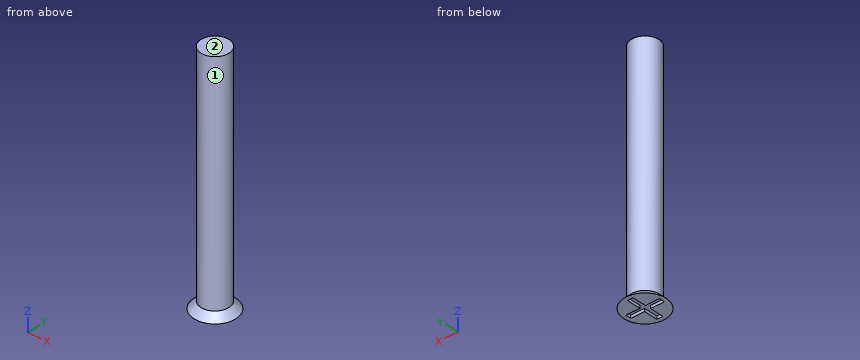
from build123d import *

# Parameters (mm, degrees)
SKETCH1_R           = 0.5
BOSS_EXTRUDE1_DEPTH = 4.1
CUT_EXTRUDE1_DEPTH  = 0.1


with BuildPart() as part:
    # Sketch1 → Boss-Extrude1 (new body, symmetric)
    with BuildSketch(Plane.XY):
        Circle(SKETCH1_R)
    extrude(amount=BOSS_EXTRUDE1_DEPTH, both=True)

    # Sketch2 → Revolve1 (revolve)
    with BuildSketch(Plane(origin=(0, 0, 0), x_dir=(0, 0, -1), z_dir=(1, 0, 0))):
        Polygon((4.35, 0.75), (4.35, 0), (4.1, 0), (4.1, 0.5), align=None)
    revolve(axis=Axis((0, 0, 2.0805), (0, 0, -1)))

    # Sketch3 → Cut-Extrude1 (cut)
    with BuildSketch(Plane(origin=(0, 0, -4.35), x_dir=(-1, 0, 0), z_dir=(0, 0, -1))):
        Polygon((0.1, 0.6), (-0.1, 0.6), (-0.1, 0.1), (-0.6, 0.1), (-0.6, -0.1), (-0.105645494, -0.1), (-0.105645494, -0.6), (0.105645494, -0.6), (0.105645494, -0.1), (0.6, -0.1), (0.6, 0.1), (0.1, 0.1), align=None)
    extrude(amount=-CUT_EXTRUDE1_DEPTH, mode=Mode.SUBTRACT)


solid = part.part
The listing builds one solid part. Answer for the finished solid, in the listing's coordinates (mm). Face numbers are marked on the shaded views. A direction names the side the tool comes from. Give positions to 0.01 mm unless a question says otherwise; leave off trailing zeros. Write each loop counter-clockwise with the first axis right and the second up, starting at its lowest first coordinate (ties: lowest second). Pieces come first, ordered by that corner, then holes.
Item 1: Which of the six approach directions +Z, -Z, +X, -X, +Y, -Y give full straight-line access (tool end or side, diameter ignored) to the marked faces 1 and 2?
Item 2: Section A-A, the plane x = 0 is taken. Write down the section's boundary in (y, z), plus the area to 3 significant figures.
Item 3: Section C-C, the plane z = 1.5 is taken. Write down the section's boundary in (x, y), plus the area to 3 significant figures.
Item 4: Find the intervals of material crossed by line 1 along Y through (x, z) = (0.05, -1.25); line 2 along Z through (x, y) = (0.05, -0.1), in increasing order.
Completed:
1. face 1: +Z
1. face 2: +Z, +X, -X, +Y, -Y
2. outline: (-0.75, -4.35) - (-0.6, -4.35) - (-0.6, -4.25) - (0.6, -4.25) - (0.6, -4.35) - (0.75, -4.35) - (0.5, -4.1) - (0.5, 4.1) - (-0.5, 4.1) - (-0.5, -4.1) - close
2. area: 8.39 mm2
3. outline: circle Ø1 at (0, 0)
3. area: 0.785 mm2
4. line 1: y = -0.5 to 0.5
4. line 2: z = -4.25 to 4.1
